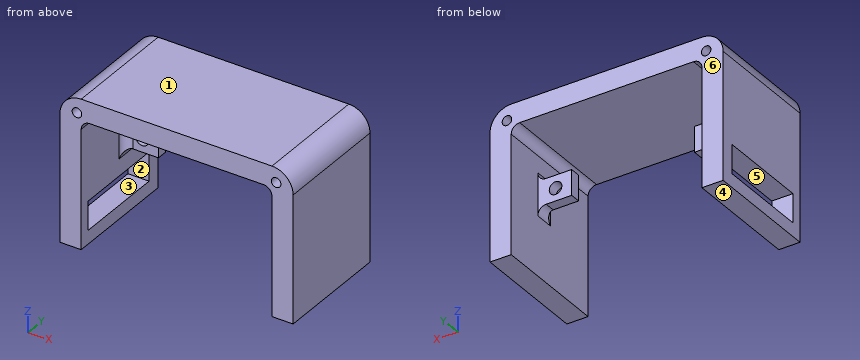
from build123d import *

# Parameters (mm, degrees)
BOSS_EXTRUDE1_DEPTH       = 31.75
SKETCH5_W                 = 7.62
SKETCH5_H                 = 3.175
BOSS_EXTRUDE2_DEPTH       = 10.16
F_6_CLEARANCE_HOLE1_D     = 3.7973
BOSS_EXTRUDE3_DEPTH       = 3.175
FILLET1_R                 = 6.35
FILLET2_R                 = 2.54
FILLET3_R                 = 2.54
FILLET4_R                 = 2.54
F_6_40_TAPPED_HOLE1_D     = 2.8702
F_6_40_TAPPED_HOLE1_DEPTH = 38.1
F_6_40_TAPPED_HOLE1_TIP   = 0.862295074
BOSS_EXTRUDE5_DEPTH       = 6.35


with BuildPart() as part:
    # Sketch1 → Boss-Extrude1 (new body)
    with BuildSketch(Plane(origin=(0, 0, 0), x_dir=(1, 0, 0), z_dir=(0, 1, 0))):
        Polygon((-34.925, -15.875), (34.925, -15.875), (34.925, 15.875), (34.925, 28.575), (28.575, 28.575), (28.575, 15.875), (28.575, -9.525), (-28.575, -9.525), (-28.575, 15.875), (-34.925, 15.875), align=None)
    extrude(amount=BOSS_EXTRUDE1_DEPTH)

    # Sketch5 → Boss-Extrude2 (add)
    with BuildSketch(Plane(origin=(-28.575, 0, 0), x_dir=(0, 0, -1), z_dir=(1, 0, 0))):
        with Locations((4.445, 18.0975)):
            Rectangle(SKETCH5_W, SKETCH5_H)
    boss_extrude2 = extrude(amount=BOSS_EXTRUDE2_DEPTH)

    # #6 Clearance Hole1 (through all)
    with Locations(Plane(origin=(0, 19.685, 0), x_dir=(1, 0, 0), z_dir=(0, 1, 0))):
        with Locations((-23.241, 4.445)):
            f_6_clearance_hole1 = Hole(F_6_CLEARANCE_HOLE1_D / 2)

    # Mirror4: Boss-Extrude2, #6 Clearance Hole1 across plane
    add(boss_extrude2.mirror(Plane(origin=(0, 0, 0), x_dir=(0, 0, 1), z_dir=(1, 0, 0))))
    add(f_6_clearance_hole1.mirror(Plane(origin=(0, 0, 0), x_dir=(0, 0, 1), z_dir=(1, 0, 0))), mode=Mode.SUBTRACT)

    # Sketch11 → Boss-Extrude3 (add)
    with BuildSketch(Plane.XZ):
        Polygon((-28.575, -28.575), (-28.575, 9.525), (28.575, 9.525), (28.575, -28.575), (34.925, -28.575), (34.925, 15.875), (-34.925, 15.875), (-34.925, -28.575), align=None)
    extrude(amount=BOSS_EXTRUDE3_DEPTH)

    # Fillet1
    fillet1_edges = [part.edges().sort_by_distance(p)[0] for p in [
        (34.925, 14.2875, 15.875),
        (-34.925, 14.2875, 15.875),
    ]]
    fillet(fillet1_edges, radius=FILLET1_R)

    # Fillet2
    fillet2_edges = [part.edges().sort_by_distance(p)[0] for p in [
        (-28.575, 18.0975, -8.255),
        (-28.575, 18.0975, -0.635),
        (28.575, 18.0975, -0.635),
        (28.575, 18.0975, -8.255),
    ]]
    fillet(fillet2_edges, radius=FILLET2_R)

    # Fillet3
    fillet3_edges = [part.edges().sort_by_distance(p)[0] for p in [
        (-28.575, 16.51, -4.445),
        (28.575, 16.51, -4.445),
    ]]
    fillet(fillet3_edges, radius=FILLET3_R)

    # Fillet4
    fillet4_edges = [part.edges().sort_by_distance(p)[0] for p in [
        (-28.575, 14.2875, 9.525),
        (28.575, 14.2875, 9.525),
    ]]
    fillet(fillet4_edges, radius=FILLET4_R)

    # #6-40 Tapped Hole1
    with Locations(Plane(origin=(0, 31.75, 0), x_dir=(1, 0, 0), z_dir=(0, 1, 0))):
        with Locations((29.845, -11.43), (-29.845, -11.43)):
            Hole(F_6_40_TAPPED_HOLE1_D / 2, depth=F_6_40_TAPPED_HOLE1_DEPTH)
            with Locations((0, 0, -(F_6_40_TAPPED_HOLE1_DEPTH + F_6_40_TAPPED_HOLE1_TIP / 2))):  # 118° drill point
                Cone(0, F_6_40_TAPPED_HOLE1_D / 2, F_6_40_TAPPED_HOLE1_TIP, mode=Mode.SUBTRACT)

    # Sketch17 → Boss-Extrude5 (add)
    with BuildSketch(Plane.ZY.offset(34.925)):
        Polygon((-28.575, 0), (-28.575, 31.75), (-15.875, 31.75), (-15.875, 27.686), (-24.511, 27.686), (-24.511, 0), align=None)
    extrude(amount=-BOSS_EXTRUDE5_DEPTH)


solid = part.part
Input: part model. Units: mm. Frame: model coordinates. Face numbers are marked on the shaded views. A direction names the side the tool comes from. Coordinates: 2 decimals unless noted, no trailing zeros. Loops run counter-clockwise (first coordinate to the right, second up) from the corner with the lowest first, then second, coordinate; pieces in that order, holes last. Notation, with made-up numbers: (59.25, -10.75) -> (112.25, -10.75) arc R21 cw to (112.25, 3.25) -> close; hole circle Ø9 at (33.5, 31.5). An arc over 180 degrees is marked (long way). Write each question's results on one line, items separated by ' | '. Start each with the question number.
Q1. Section A-A, the plane y = 1.5. Return the cut outline in (x, z) (3 decimals), plus the area to 3 significant figures.
Q2. Section D-D, the plane z = -17.5. Return the cut outline in (x, y) (3 decimals), plus the area to 3 significant figures.
Q3. Pin query (flat end, axial travel): pin 1 (6 mm diameter, centred on x = -23.241, z = -4.445, fed in from -Y); pin 2 (4.5 mm diameter, centred on x = 23.241, z = -4.445, fed in from +Y) (3 decimals); pin 3 (8.5 mm diameter, centred on x = -22.5, z = -3, fed in from -Y); pin 4 (6 mm diameter, centred on x = -27.5, z = -1, fed in from +Y). Return the tip coordinate at first contact, or that it passes through.
Q4. Ray query, line 1 (X direction, y = 13, z = 5) (3 decimals); line 2 (X direction, y = 5, z = 11.43); line 3 (X direction, y = 15, z = 11). Return the intervals inside material, ascending. Write a range as from..to.
Q5. Section C-C, the plane x = -27.5. Return the cut outline in (y, z) (3 decimals), plus the area to 3 significant figures.
Q6. Section B-B, the plane z = -7.5. Return the cut outline in (x, y) (3 decimals).
Q7. Reachability of the marked faces 1 and 2 from +Z, -Z, +X, -X, +Y, -Y: full face, straight path, thin tool, end or side. Return the list, or none.
Q8. Pull-direction query (Y, two-part tool) for the marked faces 3, 4, 5 and 6; classes: released by +Y, released by -Y, zero draft, split by the parting line, or undercut.
Found:
1) outline: (-34.925, -28.575) -> (-28.575, -28.575) -> (-28.575, -24.511) -> (-34.925, -24.511) -> close; (-34.925, -15.875) -> (-28.575, -15.875) -> (-28.575, 6.985) arc R2.54 cw to (-26.035, 9.525) -> (26.035, 9.525) arc R2.54 cw to (28.575, 6.985) -> (28.575, -28.575) -> (34.925, -28.575) -> (34.925, 9.525) arc R6.35 ccw to (28.575, 15.875) -> (-28.575, 15.875) arc R6.35 ccw to (-34.925, 9.525) -> close; hole circle Ø2.87 at (-29.845, 11.43); hole circle Ø2.87 at (29.845, 11.43) | area: 845 mm2
2) outline: (-34.925, -3.175) -> (-28.575, -3.175) -> (-28.575, 0) -> (-34.925, 0) -> close; (-34.925, 27.686) -> (-28.575, 27.686) -> (-28.575, 31.75) -> (-34.925, 31.75) -> close; (28.575, -3.175) -> (34.925, -3.175) -> (34.925, 31.75) -> (28.575, 31.75) -> close | area: 268 mm2
3) pin 1: y = 16.5 | pin 2: y = 19.685 | pin 3: y = 16.41 | pin 4: y = 31.75
4) line 1: -34.925..-28.575, 28.575..34.925 | line 2: -34.63..-31.28, -28.41..28.41, 31.28..34.63 | line 3: -34.75..-31.21, -28.48..28.48, 31.21..34.75
5) outline: (-3.175, 9.06) -> (31.75, 9.06) -> (31.75, 15.875) -> (-3.175, 15.875) -> close; (16.045, -8.72) -> (19.685, -8.72) -> (19.685, -0.17) -> (16.045, -0.17) -> close | area: 269 mm2
6) outline: (-34.925, -3.175) -> (-28.575, -3.175) -> (-28.575, 13.97) arc R2.54 cw to (-26.035, 16.51) -> (-18.415, 16.51) -> (-18.415, 19.685) -> (-28.575, 19.685) -> (-28.575, 31.75) -> (-34.925, 31.75) -> close; (18.415, 16.51) -> (26.035, 16.51) arc R2.54 cw to (28.575, 13.97) -> (28.575, -3.175) -> (34.925, -3.175) -> (34.925, 31.75) -> (28.575, 31.75) -> (28.575, 19.685) -> (18.415, 19.685) -> close
7) face 1: +Z, +X, -X, +Y, -Y | face 2: -X
8) face 3: undercut | face 4: zero draft | face 5: undercut | face 6: released by +Y
